The listing builds one solid part. Answer for the finished solid, in the listing's coordinates (mm). A direction names the side the tool comes from. Give positions to 0.01 mm unless a question says otherwise; leave off trailing zeros. Loops run counter-clockwise (first coordinate to the right, second up) from the corner with the lowest first, then second, coordinate; pieces in that order, holes last. Notation, with made-up numbers: M 26.5,56 L 54.5,56 A25 cw 54.5,74 Z; hole C 13,69 d8. An arc over 180 degrees is marked long. Use one line per item in the form item = value. Start each with the question number.
1. Straight lines are drawn through the part: line 1 (Y direction, x = 16, z = -1); line 2 (X direction, y = 2.5, z = -1.2); line 3 (X direction, y = -3.25, z = 2.2). For each, find the intervals that lie inside material, in ascending order. Write a range as from..to.
2. The part is cut by section C-C (y = 0). Write down the section's boundary in (x, z), and give its area (3 significant figures).
3. The part is cut by section B-B (z = 2). Write down the section's boundary in (x, y), and give its area (3 significant figures).
4. The mould has two halves that part along Y. Classify faces 4 (the face through (14.9, -3.5, 2.5)), 5 (the face through (15, 4, 0)), 6 (the face through (13.265, 0, -2)): released by +Y, released by -Y, zero draft, split by the parting line, or undercut.
5. Each of these flat-tipped pins is pushed along its axis until it touches: pin 1 Ø0.8 at (x, y) = (14.5, -3.5) entering from +Z; pin 2 Ø1.5 at (x, z) = (-7, 1) entering from -Y; pin 3 Ø1.1 at (y, z) = (0, -2) entering from +X. Where does it stop, or does it pass through?
6. The part is cut by section D-D (z = 0). Write down the section's boundary in (x, y), and give its area (3 significant figures).
7. For faces 1 (the face through (-15, 4, 0)), 2 (the face through (-13.265, 0, 0)), 3 (the face through (16, -3, -1)), determine the directions among +Z, -Z, +X, -X, +Y, -Y from which every point of the face is accessible in a straight line to the end or side of a thin tool.
8. The part is cut by section A-A (y = -2.25). Write down the section's boundary in (x, z), and give its area (3 significant figures).
from build123d import *

# Parameters (mm, degrees)
F0_R     = 1.5
F1_DEPTH = 12.5
F3_DEPTH = 2.5
F6_DEPTH = 3


with BuildPart() as f1:
    # F0 (on Right) → F1 (new body)
    with BuildSketch(Plane.YZ):
        Circle(F0_R)
    extrude(amount=-F1_DEPTH)

    # F2 (on Top) → F3 (join, symmetric)
    with BuildSketch(Plane.XY):
        Polygon((-12.5, -4), (-12.5, 4), (-17.26534, 4), (-17.26534, 3), (-13.26534, 3), (-13.26534, -3), (-17.26534, -3), (-17.26534, -4), align=None)
    extrude(amount=F3_DEPTH, both=True)

    # F4: F1 across plane


with BuildPart() as f1_1:
    add(f1.part)
    add(f1.part.mirror(Plane.YZ))

    # F5 (on Front) → F6 (join, symmetric)
    with BuildSketch(Plane.XZ):
        Polygon((15.386751, 2.518649), (12.5, 2.518649), (12.5, -2.481351), align=None)
    extrude(amount=F6_DEPTH, both=True)


solid = f1_1.part
Derived:
q1.line_1 = -4..-3, 3..4
q1.line_2 = -13.27..-12.5, 12.5..13.27
q1.line_3 = -17.27..-12.5, 12.5..17.27
q2.outline = M -13.27,-2.5 L -12.5,-2.5 L -12.5,-1.5 L 12.5,-1.5 L 12.5,-2.5 L 13.27,-2.5 L 13.27,-1.16 L 15.39,2.52 L 12.5,2.52 L 12.5,1.5 L -12.5,1.5 L -12.5,2.5 L -13.27,2.5 Z
q2.area = 86.6 mm2
q3.outline = M -17.27,-4 L -12.5,-4 L -12.5,4 L -17.27,4 L -17.27,3 L -13.27,3 L -13.27,-3 L -17.27,-3 Z; M 12.5,-4 L 17.27,-4 L 17.27,-3 L 15.09,-3 L 15.09,3 L 17.27,3 L 17.27,4 L 12.5,4 Z
q3.area = 39.2 mm2
q4.face_4 = zero draft
q4.face_5 = released by +Y
q4.face_6 = undercut
q5.pin_1 = 2.5
q5.pin_2 = -1.48
q5.pin_3 = 13.27
q6.outline = M -17.27,-4 L -12.5,-4 L -12.5,-1.5 L 12.5,-1.5 L 12.5,-4 L 17.27,-4 L 17.27,-3 L 13.93,-3 L 13.93,3 L 17.27,3 L 17.27,4 L 12.5,4 L 12.5,1.5 L -12.5,1.5 L -12.5,4 L -17.27,4 L -17.27,3 L -13.27,3 L -13.27,-3 L -17.27,-3 Z
q6.area = 107 mm2
q7.face_1 = +Z, -Z, +X, -X, +Y
q7.face_2 = +Z, -Z, -X
q7.face_3 = -Z, +X
q8.outline = M -13.27,-2.5 L -12.5,-2.5 L -12.5,2.5 L -13.27,2.5 Z; M 12.5,-2.5 L 13.27,-2.5 L 13.27,-1.16 L 15.39,2.52 L 12.5,2.52 Z
q8.area = 11.6 mm2
